```python
from build123d import *

# Parameters (mm, degrees)
SKETCH_1_R      = 32
EXTRUDE_2_DEPTH = 5
SKETCH_5_R      = 5


with BuildPart() as part:
    # 草图1 → 凸台-拉伸2 (new body)
    with BuildSketch(Plane.XY):
        Circle(SKETCH_1_R)
    extrude(amount=-EXTRUDE_2_DEPTH)

    # 扫描1: sweep along a path in 草图2
    with BuildLine(Plane(origin=(0, 0, 0), x_dir=(0, 0, -1), z_dir=(1, 0, 0))) as sweep_1_path:
        Line((5, 0), (15, 0))
        Line((15, 0), (15, 250))
        Line((15, 250), (25, 250))
    # 草图5 → 扫描1 (sweep)
    with BuildSketch(Plane.XY.offset(-5)):
        Circle(SKETCH_5_R)
    sweep(path=sweep_1_path.line, transition=Transition.RIGHT)


solid = part.part
```
The listing builds one solid part. Answer for the finished solid, in the listing's coordinates (mm). A direction names the side the tool comes from. Give positions to 0.01 mm unless a question says otherwise; leave off trailing zeros. Loops run counter-clockwise (first coordinate to the right, second up) from the corner with the lowest first, then second, coordinate; pieces in that order, holes last. Notation, with made-up numbers: (-7.5, 60.5) - (42.5, 60.5) arc R21 cw to (42.5, 92.5) - close; hole circle Ø4 at (60, 79). An arc over 180 degrees is marked (long way). Return JSON: item names as keys, results as strings. Group by question number.
1. Which of the six approach directions +Z, -Z, +X, -X, +Y, -Y give full straight-line access (tool end or side, diameter ignored) to faces 1 (the flat face through (0, 250, -25)), 2 (the cylindrical face through (-1.08, 126.82, -10.12)), 3 (the cylindrical face through (-1.08, 254.88, -19.27))?
2. Given pin 1 Ø12 at (y, z) = (216.5, -15) entering from -X; pin 2 Ø6 at (y, z) = (59, -7.5) entering from +X; pin 3 Ø12 at (x, z) = (4.5, -18) entering from -Y, each flat-ended and moving along its own axis, determine where each tip first touches the part or whether it passes through.
3. Find section B-B (x = 0). Write down the section's boundary in (y, z), then the cut area to 3 significant figures.
4. Find section A-A (y = 0). Write down the section's boundary in (x, z), then the cut area to 3 significant figures.
5. Find section D-D (y = 250). Write down the section's boundary in (x, z).
6. Find section C-C (z = -15). Write down the section's boundary in (x, y).
7. Straight lines are drawn through the part: line 1 (X direction, y = 0.5, z = -12.75); line 2 (Z direction, x = 13, y = 12); line 3 (Z direction, x = -3, y = 5). For each, find the intervals that lie inside material, in ascending order. Write a range as [from, to].
8. Determine the mould class of faces 4 (the cylindrical face through (-6.94, -31.24, -2.46)), 5 (the cylindrical face through (-0.651, -4.957, -10.938)), 6 (the flat face through (0, 0, 0)) for opening direction Z: pulls with the +Z half, pulls with the -Z half, needs draft (parallel to the pull), parting line crosses it, or undercut.
Verdict:
{
 "1": {"face 1": "-Z, +X, -X, +Y, -Y", "face 2": "none", "face 3": "-Z"},
 "2": {"pin 1": "stops at x = -5", "pin 2": "stops at x = 2.18", "pin 3": "stops at y = -5"},
 "3": {"outline": "(-32, -5) - (-5, -5) - (-5, -20) - (245, -20) - (245, -25) - (255, -25) - (255, -10) - (5, -10) - (5, -5) - (32, -5) - (32, 0) - (-32, 0) - close", "area": "3,020 mm^2"},
 "4": {"outline": "(-32, -5) - (-5, -5) - (-5, -15) arc R5 ccw to (5, -15) - (5, -5) - (32, -5) - (32, 0) - (-32, 0) - close", "area": "459 mm^2"},
 "5": {"outline": "(-5, -25) - (5, -25) - (5, -15) arc R5 ccw to (-5, -15) - close"},
 "6": {"outline": "(-5, 0) arc R5 ccw to (5, 0) - (5, 250) arc R5 ccw to (-5, 250) - close"},
 "7": {"line 1": "x = [-4.97, 4.97]", "line 2": "z = [-5, 0]", "line 3": "z = [-19, -11], [-5, 0]"},
 "8": {"face 4": "needs draft", "face 5": "undercut", "face 6": "pulls with the +Z half"}
}
